Autodesk Inventor part; units mm, degrees
ref_plane "YZ Plane" through (0, 0, 0) normal (1, 0, 0) x (0, 1, 0)
ref_plane "XZ Plane" through (0, 0, 0) normal (0, 1, 0) x (-1, 0, 0)
ref_plane "XY Plane" through (0, 0, 0) normal (0, 0, 1) x (1, 0, 0)
sketch "스케치1" plane through (0, 0, 0) normal (0, 0, 1) x (1, 0, 0)
  line L0 (0, 0) -> (-20, 0)
  line L1 (-20, 0) -> (-20, 40)
  line L2 (-20, 40) -> (0, 40)
  line L3 (0, 40) -> (0, 0)
  circle A0 centre (-20, 20) radius 6.25
  point P0 (-20, 26.25)
  point P1 (-20, 13.75)
  dimension "d0" = 40
  dimension "d1" = 20
  dimension "d2" = 20
  dimension "d3" = 12.5
extrude "돌출1" add sketch "스케치1" along normal blind 118 contours L0 L1 A0 L2 L3
sketch "스케치2" plane through (0, 0, 118) normal (0, 0, 1) x (1, 0, 0)
  line L0 (-20, 40) -> (-20, 26.25)
  line L1 (-20, 36) -> (-4, 36)
  line L2 (-4, 36) -> (-4, 4)
  line L3 (-4, 4) -> (-20, 4)
  line L4 (-20, 13.75) -> (-20, 0)
  line L5 (0, 40) -> (-20, 40)
  point P0 (0, 0)
  dimension "d6" = 16
  dimension "d7" = 32
  dimension "d8" = 4
sketch "스케치3" plane through (0, 0, 118) normal (0, 0, 1) x (1, 0, 0)
  line L0 (-20, 36) -> (-4, 36)
  line L1 (-4, 36) -> (-4, 4)
  line L2 (-4, 4) -> (-20, 4)
  line L3 (-20, 13.75) -> (-20, 0)
  line L4 (-20, 40) -> (-20, 26.25)
  point P0 (0, 0)
sketch "스케치4" plane through (0, 0, 118) normal (0, 0, 1) x (1, 0, 0)
  line L0 (-20, 40) -> (-20, 26.25)
  line L1 (-20, 35.8924) -> (-20, 26.25)
  line L2 (-20, 13.75) -> (-20, 0)
  line L3 (-20, 4.1853) -> (-20, 13.75)
  point P0 (0, 0)
sketch "스케치5" plane through (0, 0, 118) normal (0, 0, 1) x (1, 0, 0)
  line L0 (-20, 36) -> (-4, 36)
  line L1 (-4, 36) -> (-4, 4)
  line L2 (-4, 4) -> (-20, 4)
  line L3 (-20, 13.75) -> (-20, 0)
  line L4 (-20, 40) -> (-20, 26.25)
  point P0 (0, 0)
  point P1 (-20, 4.1853)
sketch "스케치6" plane through (0, 0, 0) normal (0, 0, -1) x (-1, 0, 0)
  line L0 (20, 13.75) -> (20, 0)
  line L1 (20, 4) -> (4, 4)
  line L2 (4, 4) -> (4, 36)
  line L3 (4, 36) -> (20, 36)
  line L4 (20, 36) -> (20, 4)
  line L5 (20, 0) -> (0, 0)
  arc A0 (20, 26.25) -> (20, 13.75) centre (20, 20) ccw
  dimension "d9" = 16
  dimension "d10" = 32
  dimension "d11" = 4
extrude "돌출2" cut sketch "스케치6" against normal blind 112 contours L0 L1 L2 L3 L4 A0
sketch "스케치8" plane through (-20, 26.25, 118) normal (-1, 0, 0) x (0, 0, 1)
  circle A0 centre (-3, 5.5) radius 2
  circle A1 centre (-3, -18) radius 2
  line L0 (0, -12.5) -> (0, -26.25)
  line L1 (-6, -12.5) -> (0, -12.5)
  line L2 (-6, 0) -> (0, 0)
  line L3 (0, 13.75) -> (0, 0)
  point P0 (-118, -26.25)
  dimension "d22" = 4
  dimension "d23" = 4
  dimension "d24" = 3
  dimension "d25" = 5.5
  dimension "d26" = 5.5
  dimension "d27" = 3
extrude "돌출4" cut sketch "스케치8" against normal blind 10
properties part number "hard_support_wm"
The model under review builds one solid part; all positions refer to its coordinate system, in mm. A direction names the side the tool comes from. Round coordinates to 2 decimals unless told otherwise and drop trailing zeros. Loops run counter-clockwise (first coordinate to the right, second up) from the corner with the lowest first, then second, coordinate; pieces in that order, holes last. Notation, with made-up numbers: M -32.75,10 L 20.25,10 A20 cw 20.25,19 Z; hole C 0.25,81.5 d8. An arc over 180 degrees is marked long. Answer as a JSON object with one key per item and string values.
Item 1: Tool access review of faces 1 (the face through (-10, 8, 115)), 2 (the face through (-10, 40, 58)), 3 (the face through (-12, 4, 55)): name each direction out of +Z, -Z, +X, -X, +Y, -Y from which nothing blocks a thin tool from reaching the whole face with its end or side.
Check sheet entries:
{"face 1": "-X", "face 2": "+Z, -Z, +X, -X, +Y", "face 3": "-Z, -X"}
Item 2: We need section C-C, the plane z = 115. State the section outline as (x, y) points.
Check sheet entries:
{"outline": "M -20,0 L 0,0 L 0,40 L -20,40 L -20,33.75 L -10,33.75 L -10,29.75 L -20,29.75 L -20,26.25 A6.25 cw -20,13.75 L -20,10.25 L -10,10.25 L -10,6.25 L -20,6.25 Z"}
Item 3: We need section A-A, the plane x = -12. State the section outline as (y, z) points, and give its area (3 significant figures).
Check sheet entries:
{"outline": "M 0,0 L 4,0 L 4,112 L 36,112 L 36,0 L 40,0 L 40,118 L 0,118 Z; hole C 8.25,115 d4; hole C 31.75,115 d4", "area": "1,110 mm2"}
Item 4: The part is to be moulded in two halves that separate along Z. For faces 4 (the face through (-12, 20, 112)), 5 (the face through (-10, 32, 115)), 6 (the face through (-15.1, 8.3, 113)), 7 (the face through (-4, 20, 55)), say which applies: +Z half, -Z half, draft (parallel to the pull), parting line (faces both ways), or undercut.
Check sheet entries:
{"face 4": "-Z half", "face 5": "undercut", "face 6": "undercut", "face 7": "draft"}
Item 5: We need section B-B, the plane y = 8.25. State the section outline as (x, z) points.
Check sheet entries:
{"outline": "M -20,112 L -4,112 L -4,0 L 0,0 L 0,118 L -20,118 L -20,117 L -10,117 L -10,113 L -20,113 Z"}
Item 6: We need section D-D, the plane x = -18. State the section outline as (y, z) points, and give its area (3 significant figures).
Check sheet entries:
{"outline": "M 0,0 L 4,0 L 4,112 L 14.08,112 L 14.08,118 L 0,118 Z; M 25.92,112 L 36,112 L 36,0 L 40,0 L 40,118 L 25.92,118 Z; hole C 8.25,115 d4; hole C 31.75,115 d4", "area": "1,040 mm2"}
Item 7: Clearance check with flat-ended pins moving along their axes: P1, Ø6.5, axis at y = 8.25, z = 115, coming from the -X side; P2, Ø12, axis at y = 25, z = 30.5, coming from the -X side; P3, Ø5, axis at x = -14.5, y = 17.5, coming from the -Z side. State where each tip first meets the part, or that it passes through.
Check sheet entries:
{"P1": "x = -20", "P2": "x = -4", "P3": "z = 112"}
Item 8: For line 1 along Y through (x, z) = (-14, 14.5); line 2 along Y through (x, z) = (-17, 115); line 3 along X through (y, z) = (7.5, 56.5), list the stretches that pass through material, from the lowest coordinate up.
Check sheet entries:
{"line 1": "0 to 4, 36 to 40", "line 2": "0 to 6.25, 10.25 to 14.52, 25.48 to 29.75, 33.75 to 40", "line 3": "-4 to 0"}
